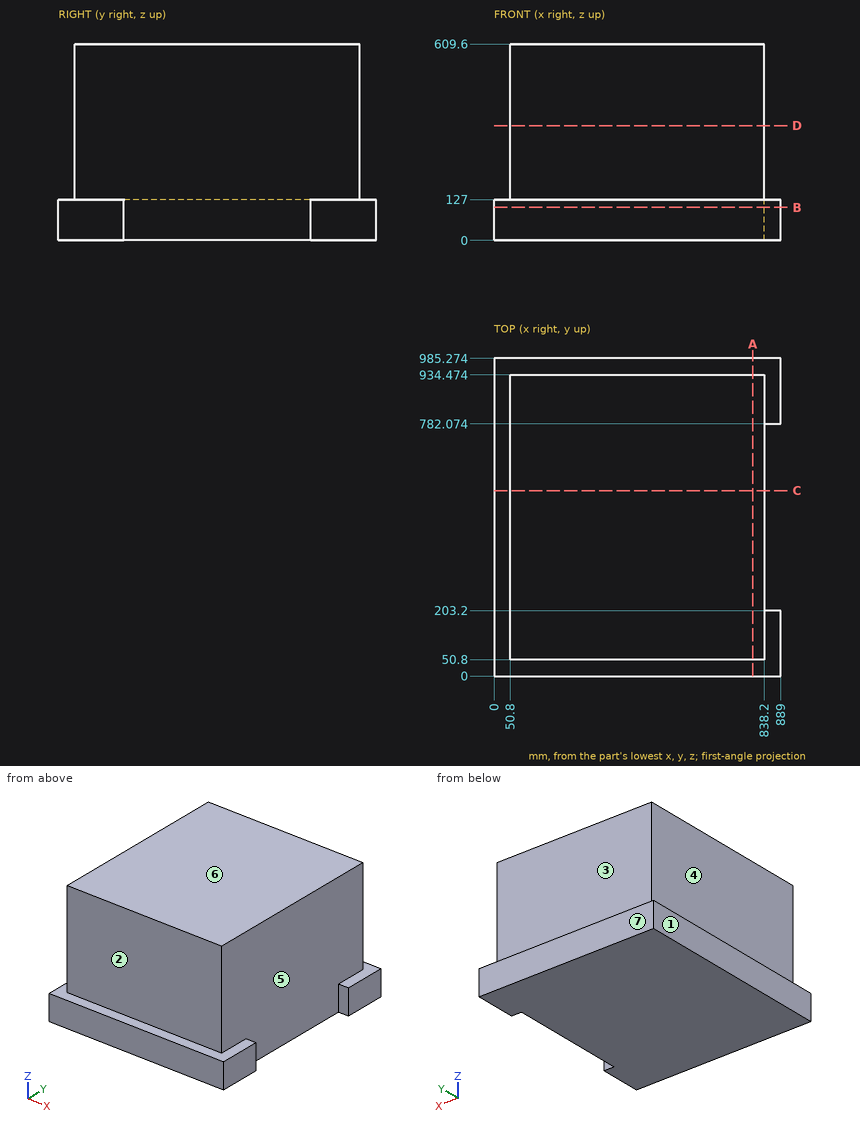
Design review of the part shown in the three views and the two pictorial views. Dimensions are in mm from the part's minimum x, y and z. A direction names the side the tool comes from. Give positions to 0.01 mm unless a question says otherwise; leave off trailing zeros. Loops run counter-clockwise (first coordinate to the right, second up) from the corner with the lowest first, then second, coordinate; pieces in that order, holes last. Notation, with made-up numbers: (19, 21.5) -> (73, 21.5) arc R13 ccw to (73, 46.5) -> close; hole circle Ø4 at (4, 84). An arc over 180 degrees is marked (long way). Put each result on its own line as item: value. Start each with the question number.
1. We need section D-D on z = 356.5. State the section outline as (x, y) points.
2. Wall thickness on probe 1 along Y at (x, z) = (824.5, 209); probe 2 along X at (y, z) = (471.5, 104); probe 3 along X at (y, z) = (726, 443): over which ranges is each line inside the solid? List them lowest first.
3. We need section C-C on y = 575. State the section outline as (x, z) points.
4. For the marked faces 1, 2, 3 and 4, list the 3-axis set-ups (+Z, -Z, +X, -X, +Y, -Y) from which the entire face can be reached by the end or side of a thin tool; tool diameter is ignored.
5. Clearance check with flat-ended pins moving along their axes: P1, Ø8, axis at x = 564.5, z = 476.5, coming from the -Y side; P2, Ø12, axis at y = 843, z = 129.5, coming from the -X side; P3, Ø3, axis at x = 337.5, z = 164.5, coming from the +Y side; P4, Ø8, axis at y = 543, z = 450, coming from the -X side. State where each tip first meets the part, or that it passes through.
6. We need section B-B on z = 102.5. State the section outline as (x, y) points, then the cut area to 4 significant figures.
7. Mouldability with a two-part tool opening along Y and no side actions: class the marked faces 5, 6 and 7 as released by +Y, released by -Y, zero draft, split by the parting line, or undercut.
8. We need section A-A on x = 803. State the section outline as (y, z) points, then the cut area to 3 significant figures.
Determined:
1. outline: (50.8, 50.8) -> (838.2, 50.8) -> (838.2, 934.47) -> (50.8, 934.47) -> close
2. probe 1: 50.8 to 934.47
2. probe 2: 0 to 838.2
2. probe 3: 50.8 to 838.2
3. outline: (0, 0) -> (838.2, 0) -> (838.2, 609.6) -> (50.8, 609.6) -> (50.8, 127) -> (0, 127) -> close
4. face 1: +Z, -Z, -X, +Y, -Y
4. face 2: +Z, +X, -X, -Y
4. face 3: +Z, +X, -X, +Y
4. face 4: +Z, -X, +Y, -Y
5. P1: y = 50.8
5. P2: x = 0
5. P3: y = 934.47
5. P4: x = 50.8
6. outline: (0, 0) -> (889, 0) -> (889, 203.2) -> (838.2, 203.2) -> (838.2, 782.07) -> (889, 782.07) -> (889, 985.27) -> (0, 985.27) -> close
6. area: 846,500 mm^2
7. face 5: undercut
7. face 6: zero draft
7. face 7: released by +Y
8. outline: (0, 0) -> (985.27, 0) -> (985.27, 127) -> (934.47, 127) -> (934.47, 609.6) -> (50.8, 609.6) -> (50.8, 127) -> (0, 127) -> close
8. area: 552,000 mm^2
